from build123d import *

# Parameters (mm, degrees)
SKETCH1_W                  = 52
SKETCH1_H                  = 55
BOSS_EXTRUDE1_DEPTH        = 50
SKETCH2_W                  = 49
SKETCH2_H                  = 52
CUT_EXTRUDE1_DEPTH         = 89.926936302
CUT_EXTRUDE2_DEPTH         = 89.926936302
CUT_EXTRUDE3_DEPTH         = 89.926936302
CUT_EXTRUDE4_DEPTH         = 89.926936302
CUT_EXTRUDE5_DEPTH         = 88.206651122
F_18_0_18_DIAMETER_HOLE1_D = 18
F_4_0_4_DIAMETER_HOLE1_D   = 4
FILLET1_R                  = 3
FILLET2_R                  = 5
BOSS_EXTRUDE2_DEPTH        = 1
BOSS_EXTRUDE3_DEPTH        = 1
BOSS_EXTRUDE4_START        = 1
BOSS_EXTRUDE4_DEPTH        = 1
BOSS_EXTRUDE5_DEPTH        = 1


with BuildPart() as part:
    # Sketch1 → Boss-Extrude1 (new body)
    with BuildSketch(Plane(origin=(50, 0, 0), x_dir=(0, 0, -1), z_dir=(1, 0, 0))):
        with Locations((-26, -24.5)):
            Rectangle(SKETCH1_W, SKETCH1_H)
    extrude(amount=-BOSS_EXTRUDE1_DEPTH)

    # Sketch2 → Cut-Extrude1 (cut, through all)
    with BuildSketch(Plane.ZY):
        with Locations((27.5, -26)):
            Rectangle(SKETCH2_W, SKETCH2_H)
    extrude(amount=-CUT_EXTRUDE1_DEPTH, mode=Mode.SUBTRACT)

    # Sketch3 → Cut-Extrude2 (cut, through all)
    with BuildSketch(Plane(origin=(0, 0, 0), x_dir=(-1, 0, 0), z_dir=(0, 0, -1))):
        with BuildLine():
            Line((-33.1, -37.9), (-38.900000611, -37.9))
            ThreePointArc((-38.900000611, -37.9), (-41.000000611, -40), (-38.900000611, -42.1))
            Line((-38.900000611, -42.1), (-33.1, -42.1))
            ThreePointArc((-33.1, -42.1), (-31, -40), (-33.1, -37.9))
        make_face()
    extrude(amount=-CUT_EXTRUDE2_DEPTH, mode=Mode.SUBTRACT)

    # Sketch4 → Cut-Extrude3 (cut, through all)
    with BuildSketch(Plane(origin=(0, 0, 0), x_dir=(-1, 0, 0), z_dir=(0, 0, -1))):
        with BuildLine():
            Line((-16.9, -14.1), (-11.1, -14.1))
            ThreePointArc((-11.1, -14.1), (-9, -12), (-11.1, -9.9))
            Line((-11.1, -9.9), (-16.9, -9.9))
            ThreePointArc((-16.9, -9.9), (-19, -12), (-16.9, -14.1))
        make_face()
    extrude(amount=-CUT_EXTRUDE3_DEPTH, mode=Mode.SUBTRACT)

    # Sketch5 → Cut-Extrude4 (cut, through all)
    with BuildSketch(Plane(origin=(0, 0, 0), x_dir=(-1, 0, 0), z_dir=(0, 0, -1))):
        with BuildLine():
            Line((-16.9, -42.1), (-11.1, -42.1))
            ThreePointArc((-11.1, -42.1), (-9, -40), (-11.1, -37.9))
            Line((-11.1, -37.9), (-16.9, -37.9))
            ThreePointArc((-16.9, -37.9), (-19, -40), (-16.9, -42.1))
        make_face()
    extrude(amount=-CUT_EXTRUDE4_DEPTH, mode=Mode.SUBTRACT)

    # Sketch6 → Cut-Extrude5 (cut, through all)
    with BuildSketch(Plane.XY.offset(3)):
        with BuildLine():
            Line((38.9, -9.9), (33.1, -9.9))
            ThreePointArc((33.1, -9.9), (31, -12), (33.1, -14.1))
            Line((33.1, -14.1), (38.9, -14.1))
            ThreePointArc((38.9, -14.1), (41, -12), (38.9, -9.9))
        make_face()
    extrude(amount=-CUT_EXTRUDE5_DEPTH, mode=Mode.SUBTRACT)

    # Ø18.0 (18) Diameter Hole1 (through all)
    with Locations(Plane(origin=(0, 0, 0), x_dir=(-1, 0, 0), z_dir=(0, -1, 0))):
        with Locations((-25, -28)):
            Hole(F_18_0_18_DIAMETER_HOLE1_D / 2)

    # Ø4.0 (4) Diameter Hole1 (through all)
    with Locations(Plane(origin=(0, 0, 0), x_dir=(-1, 0, 0), z_dir=(0, -1, 0))):
        with Locations((-10.5, -28), (-39.5, -28)):
            Hole(F_4_0_4_DIAMETER_HOLE1_D / 2)

    # Fillet1
    fillet1_edges = [part.edges().sort_by_distance(p)[0] for p in [
        (25, 3, 0),
    ]]
    fillet(fillet1_edges, radius=FILLET1_R)

    # Fillet2
    fillet2_edges = [part.edges().sort_by_distance(p)[0] for p in [
        (50, -52, 1.5),
        (0, -52, 1.5),
        (0, 1.5, 52),
        (50, 1.5, 52),
    ]]
    fillet(fillet2_edges, radius=FILLET2_R)

    # Sketch12 → Boss-Extrude2 (add)
    with BuildSketch(Plane.ZY):
        Polygon((3, -47), (47, 0), (3, 0), align=None)
    extrude(amount=-BOSS_EXTRUDE2_DEPTH)

    # Sketch13 → Boss-Extrude3 (add)
    with BuildSketch(Plane(origin=(50, 0, 0), x_dir=(0, 0, -1), z_dir=(1, 0, 0))):
        Polygon((-3, -47), (-3, 0), (-47, 0), align=None)
    extrude(amount=-BOSS_EXTRUDE3_DEPTH)

    # Sketch14 → Boss-Extrude4 (add)
    with BuildSketch(Plane.ZY.offset(BOSS_EXTRUDE4_START)):
        with BuildLine():
            Line((0, 0), (0, -47))
            Line((0, -47), (3, -47))
            Line((3, -47), (47, 0))
            Line((47, 0), (47, 3))
            Line((47, 3), (3, 3))
            ThreePointArc((3, 3), (0.878679656, 2.121320344), (0, 0))
        make_face()
    extrude(amount=-BOSS_EXTRUDE4_DEPTH)

    # Sketch15 → Boss-Extrude5 (add)
    with BuildSketch(Plane(origin=(50, 0, 0), x_dir=(0, 0, -1), z_dir=(1, 0, 0))):
        with BuildLine():
            Line((-3, 3), (-47, 3))
            Line((-47, 3), (-47, 0))
            Line((-47, 0), (-3, -47))
            Line((-3, -47), (0, -47))
            Line((0, -47), (0, 0))
            ThreePointArc((0, 0), (-0.878679656, 2.121320344), (-3, 3))
        make_face()
    extrude(amount=BOSS_EXTRUDE5_DEPTH)


solid = part.part
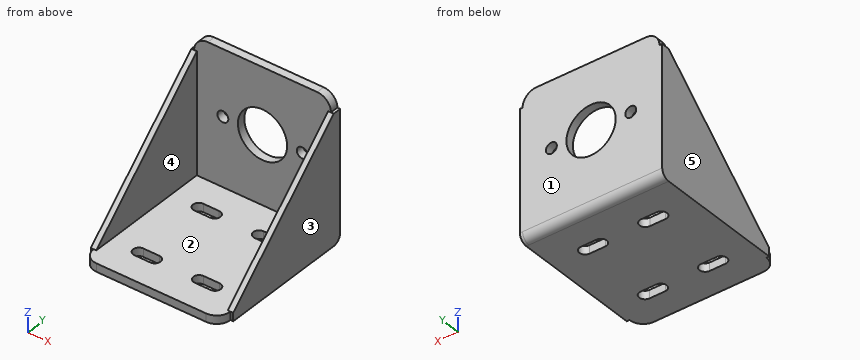
Read the model definition and answer for the solid it produces. Units are mm, in the model's axes. Face numbers are marked on the shaded views. A direction names the side the tool comes from. Give positions to 0.01 mm unless a question says otherwise; leave off trailing zeros. Write each loop counter-clockwise with the first axis right and the second up, starting at its lowest first coordinate (ties: lowest second). Pieces come first, ordered by that corner, then holes. Notation, with made-up numbers: (-0.75, 13.5) - (13.25, 13.5) arc R25 cw to (13.25, 51.5) - close; hole circle Ø1 at (44.25, -22.5). An arc over 180 degrees is marked (long way). Answer in a Markdown table with one row per item. Add a question column.
Item 1: Determine the mould class of the marked faces 3, 4 and 5 for opening direction X: pulls with the +X half, pulls with the -X half, needs draft (parallel to the pull), parting line crosses it, or undercut.
Item 2: Section A-A, the plane y = -12 is taken. Write down the section's boundary in (x, z), and give its area (3 significant figures).
Item 3: Find the intervals of material crossed by L1, parallel to X at y = -4.5, z = 11; L2, parallel to Z at x = 8, y = -41, in increasing order.
Item 4: Section D-D, the plane x = 40 is taken. Write down the section's boundary in (y, z), and give its area (3 significant figures).
Item 5: Flat-ended cylindrical pins translate along their axes: P1, Ø0.8, axis at x = -0.5, z = 2, coming from the -Y side; P2, Ø1.5, axis at x = 34.5, z = 1.5, coming from the +Y side; P3, Ø0.9, axis at x = 36.5, z = 1.5, coming from the +Y side. Find the tip coordinate at first contact, or state that the pin passes through.
Item 6: Section C-C, the plane z = 33.5 is taken. Write down the section's boundary in (x, y).
Item 7: Section B-B, the plane x = 23 is taken. Write down the section's boundary in (y, z).
Item 8: A tool of negligible diameter and unlimited length cuts with its end or side. For the marked faces 1 and 2, from which of +Z, -Z, +X, -X, +Y, -Y can it reach the whole face along a straight path? Write none if from no direction.
Recorded:
| question | item | result |
|---|---|---|
| 1 | face 3 | pulls with the +X half |
| 1 | face 4 | undercut |
| 1 | face 5 | pulls with the -X half |
| 2 | outline | (-1, 0) - (9, 0) - (9, 3) - (1, 3) - (1, 35.77) - (-1, 35.77) - close; (19, 0) - (31, 0) - (31, 3) - (19, 3) - close; (41, 0) - (51, 0) - (51, 35.77) - (49, 35.77) - (49, 3) - (41, 3) - close |
| 2 | area | 227 mm2 |
| 3 | L1 | x = -1 to 1, 49 to 51 |
| 3 | L2 | z = 0 to 3 |
| 4 | outline | (-52, 0) - (-41.79, 0) - (-41.79, 3) - (-52, 3) - close; (-38.21, 0) - (-13.79, 0) - (-13.79, 3) - (-38.21, 3) - close; (-10.21, 0) - (0, 0) arc R3 ccw to (3, 3) - (3, 26.06) - (0, 26.06) - (0, 3) - (-10.21, 3) - close; (0, 29.94) - (3, 29.94) - (3, 52) - (0, 52) - close |
| 4 | area | 277 mm2 |
| 5 | P1 | stops at y = -47 |
| 5 | P2 | stops at y = 2.9 |
| 5 | P3 | stops at y = 2.81 |
| 6 | outline | (-1, -14.42) - (1, -14.42) - (1, 0) - (17.88, 0) - (17.88, 3) - (-1, 3) - close; (32.12, 0) - (49, 0) - (49, -14.42) - (51, -14.42) - (51, 3) - (32.12, 3) - close |
| 7 | outline | (-52, 0) - (0, 0) arc R3 ccw to (3, 3) - (3, 19.23) - (0, 19.23) - (0, 3) - (-52, 3) - close; (0, 36.77) - (3, 36.77) - (3, 52) - (0, 52) - close |
| 8 | face 1 | +Z, -Z, +X, -X, +Y |
| 8 | face 2 | +Z, -Y |
